The drawing under review shows one solid part. Ordinate dimensions are in mm from its lowest x, y, z. A direction names the side the tool comes from. Coordinates: 2 decimals unless noted, no trailing zeros. Loops run counter-clockwise (first coordinate to the right, second up) from the corner with the lowest first, then second, coordinate; pieces in that order, holes last. Notation, with made-up numbers: M 26,57.25 L 37,57.25 A32 ccw 37,94.25 Z; hole C -35.75,-8 d7. An arc over 180 degrees is marked long. Use one line per item in the form item = value.
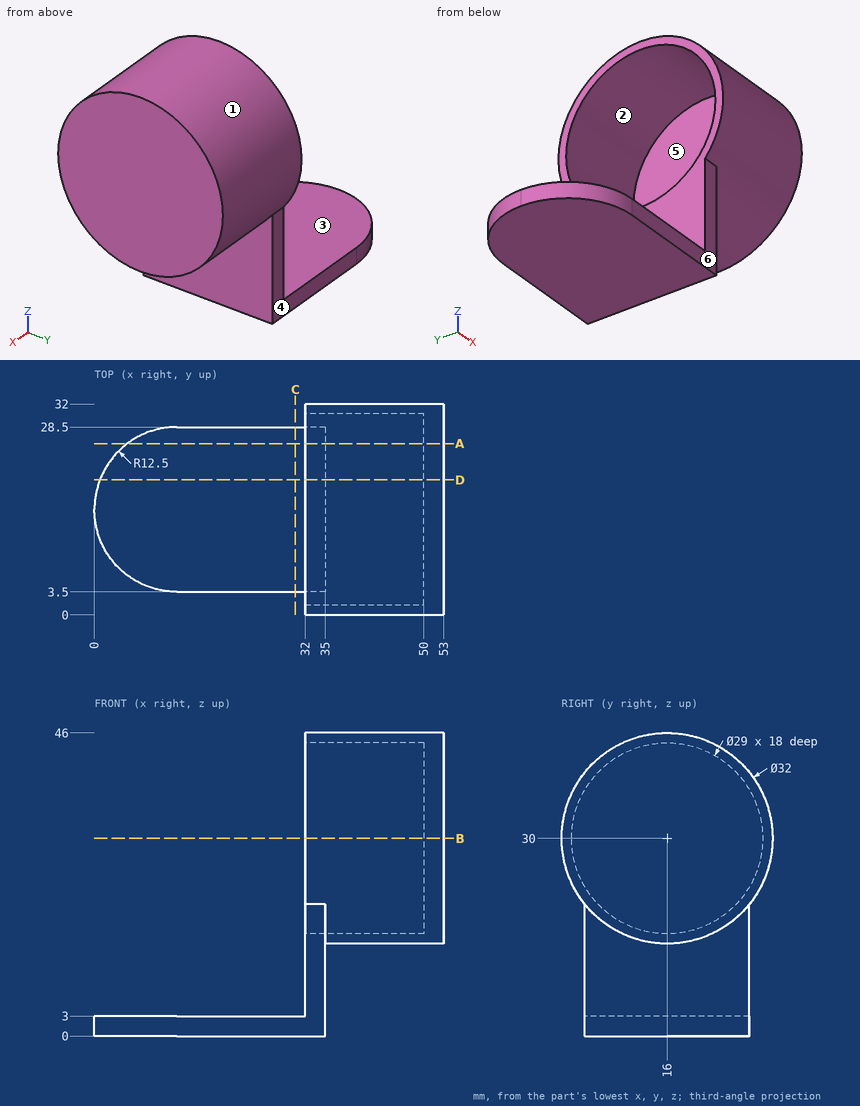
1. Consider section D-D on y = 20.5. Write out the cut boundary in (x, z).
Computed values:
outline = M 0.84,0 L 35,0 L 35,14.65 L 53,14.65 L 53,45.35 L 32,45.35 L 32,43.78 L 50,43.78 L 50,16.22 L 32,16.22 L 32,3 L 0.84,3 Z
2. Draft analysis for pull direction Y (two halves, no side actions). For the marked faces 1, 2 and 3, state which applies: +Y half, -Y half, draft (parallel to the pull), parting line (faces both ways), or undercut.
Computed values:
face_1 = parting line
face_2 = undercut
face_3 = draft
3. Tool access review of the marked faces 4, 5 and 6: name each direction out of +Z, -Z, +X, -X, +Y, -Y from which nothing blocks a thin tool from reaching the whole face with its end or side.
Computed values:
face_4 = -Z, +X, -X, +Y
face_5 = -X
face_6 = -Z, +X, -X, -Y
4. Wall thickness on line 1 along Z through (x, y) = (35.75, 16); line 2 along X through (y, z) = (20.5, 21); line 3 along Z through (x, y) = (15, 6): over which ranges is each line inside the solid? List them lowest first. Write a range as from..to.
Computed values:
line_1 = 14..15.5, 44.5..46
line_2 = 50..53
line_3 = 0..3
5. Consider section B-B on z = 30. Write out the cut boundary in (x, y), plus the area to 3 significant figures.
Computed values:
outline = M 32,0 L 53,0 L 53,32 L 32,32 L 32,30.5 L 50,30.5 L 50,1.5 L 32,1.5 Z
area = 150 mm2
6. Consider section A-A on y = 26. Write out the cut boundary in (x, z), plus the area to 3 significant figures.
Computed values:
outline = M 5,0 L 35,0 L 35,17.51 L 53,17.51 L 53,42.49 L 32,42.49 L 32,40.5 L 50,40.5 L 50,19.5 L 32,19.5 L 32,3 L 5,3 Z
area = 280 mm2
7. Consider section C-C on x = 30.5. Write out the cut boundary in (y, z), plus the area to 3 significant figures.
Computed values:
outline = M 3.5,0 L 28.5,0 L 28.5,3 L 3.5,3 Z
area = 75.0 mm2
8. For pin 1 Ø9.5 at (y, z) = (18, 19) entering from -X; pin 2 Ø10 at (x, y) = (47, 22.5) entering from -Z; pin 3 Ø3 at (x, y) = (41.5, 22.5) entering from -Z, all flat-tipped, find the tip position at first contact; note any pin that passes through.
Computed values:
pin_1 = 32
pin_2 = 14.07
pin_3 = 14.8
